Here's the drawing with two shaded views (mm, measured from the low corner). I have some questions. A direction names the side the tool comes from. Round coordinates to 2 decimals unless told otherwise and drop trailing zeros. Loops run counter-clockwise (first coordinate to the right, second up) from the corner with the lowest first, then second, coordinate; pieces in that order, holes last.
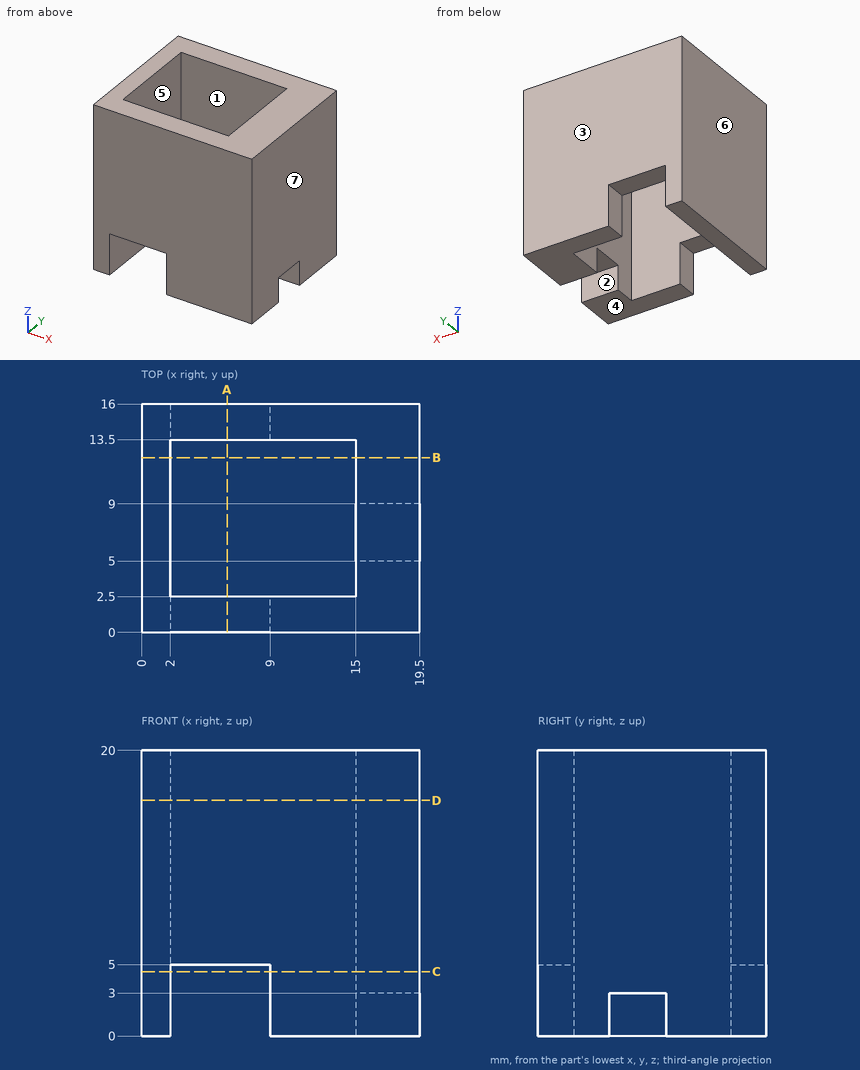
(1) If we section it at A-A, the plane x = 6: List the corners of the cut face in (y, z) for me.
Worked answers:
outline: (0, 5) - (2.5, 5) - (2.5, 20) - (0, 20) - close; (13.5, 5) - (16, 5) - (16, 20) - (13.5, 20) - close
(2) If we mould it in two halves opening along X, with no side actions, what happens to the marked faces 4, 5, 6 and 7? For each: released by +X, released by -X, zero draft, split by the parting line, or undercut.
Worked answers:
face 4: zero draft
face 5: undercut
face 6: released by -X
face 7: released by +X
(3) If we section it at C-C, the plane z = 4.5: List the corners of the cut face in (x, y) for me, then the cut area to 3 significant figures.
Worked answers:
outline: (0, 0) - (2, 0) - (2, 16) - (0, 16) - close; (9, 0) - (19.5, 0) - (19.5, 16) - (9, 16) - (9, 13.5) - (15, 13.5) - (15, 2.5) - (9, 2.5) - close
area: 134 mm2
(4) For the marked faces 1, 2 and 3, which set-ups out of +Z, -Z, +X, -X, +Y, -Y let a thin tool reach every point of the face, with its end or its side?
Worked answers:
face 1: +Z, -Z
face 2: -Z, +X
face 3: +Z, -Z, +X, -X, +Y
(5) If we section it at B-B, the plane y = 12.25: List the corners of the cut face in (x, z) for me.
Worked answers:
outline: (0, 0) - (2, 0) - (2, 20) - (0, 20) - close; (15, 0) - (19.5, 0) - (19.5, 20) - (15, 20) - close
(6) Will this pin go through, and if not, where does the flat tip stop? P1, Ø1.2, axis at x = 7, y = 1.5, coming from the -Z side.
Worked answers:
P1: stops at z = 5
(7) If I drill on line 1 (X direction, y = 3, z = 12); line 2 (Y direction, x = 7, z = 10.5); line 3 (Z direction, x = 18, y = 6.5), over which ranges is the centre line in solid material (lowest first)?
Worked answers:
line 1: x = 0 to 2, 15 to 19.5
line 2: y = 0 to 2.5, 13.5 to 16
line 3: z = 3 to 20
(8) If we section it at D-D, the plane z = 16.5: List the corners of the cut face in (x, y) for me.
Worked answers:
outline: (0, 0) - (19.5, 0) - (19.5, 16) - (0, 16) - close; hole (2, 2.5) - (15, 2.5) - (15, 13.5) - (2, 13.5) - close
